For this review, take the finished solid that the model builds, in its own axes (mm). A direction names the side the tool comes from. Round coordinates to 2 decimals unless told otherwise and drop trailing zeros. Loops run counter-clockwise (first coordinate to the right, second up) from the corner with the lowest first, then second, coordinate; pieces in that order, holes last.
```python
from build123d import *

# Parameters (mm, degrees)
ESQUISSE1_R             = 20
BOSS_EXTRU_1_DEPTH      = 85
ESQUISSE6_R             = 8
ENL_V_MAT_EXTRU_1_DEPTH = 85
ESQUISSE7_R             = 11
ENL_V_MAT_EXTRU_2_DEPTH = 7
ESQUISSE11_W            = 3
ESQUISSE11_H            = 2


with BuildPart() as part:
    # Esquisse1 → Boss.-Extru.1 (new body)
    with BuildSketch(Plane(origin=(0, 0, 0), x_dir=(1, 0, 0), z_dir=(0, 1, 0))):
        with Locations(Location((0, 0, 0), (0, 0, 270))):
            Circle(ESQUISSE1_R)
    extrude(amount=BOSS_EXTRU_1_DEPTH)

    # Esquisse6 → Enlèv. mat.-Extru.1 (cut)
    with BuildSketch(Plane.XZ):
        with Locations(Location((0, 0, 0), (0, 0, 270))):
            Circle(ESQUISSE6_R)
    extrude(amount=-ENL_V_MAT_EXTRU_1_DEPTH, mode=Mode.SUBTRACT)

    # Esquisse7 → Enlèv. mat.-Extru.2 (cut)
    with BuildSketch(Plane.XZ):
        with Locations(Location((0, 0, 0), (0, 0, 270))):
            Circle(ESQUISSE7_R)
    enl_v_mat_extru_2 = extrude(amount=-ENL_V_MAT_EXTRU_2_DEPTH, mode=Mode.SUBTRACT)

    # Symétrie1: Enlèv. mat.-Extru.2 across plane
    add(enl_v_mat_extru_2.mirror(Plane.ZX.offset(42.5)), mode=Mode.SUBTRACT)

    # Esquisse11 → Révolution1 (revolve)
    with BuildSketch(Plane(origin=(0, 0, 0), x_dir=(0, 0, -1), z_dir=(1, 0, 0))):
        with Locations((21.485433731, 1)):
            Rectangle(ESQUISSE11_W, ESQUISSE11_H)
    r_volution1 = revolve(axis=Axis((0, 85, 0), (0, -1, 0)))

    # Symétrie2: Révolution1 across plane
    add(r_volution1.mirror(Plane.ZX.offset(42.5)))


solid = part.part
```
(1) For faces 1 (the cylindrical face through (15.535, 83.986, 16.941)), 2 (the flat face through (-20.3, 83, -1.8)), 3 (the cylindrical face through (-10.74, 3.45, 2.38)), 4 (the cylindrical face through (-10.74, 81.55, 2.38)), list the 3-axis set-ups (+Z, -Z, +X, -X, +Y, -Y) from which the entire face can be reached by the end or side of a thin tool; tool diameter is ignored.
(2) Add section C-C (y = 6). Give the boundary of the cut face in (x, z), plus the area to 3 significant figures.
(3) Add section D-D (z = -9.5). Give the boundary of the cut face in (x, y).
(4) Add section A-A (x = 0). Give the boundary of the cut face in (y, z).
(5) The part is to be moulded in two halves that separate along Z. For faces 5 (the flat face through (-8, 78, 2)), 6 (the flat face through (-10, 85, -5)), 7 (the cylindrical face through (-19.524, 41.933, -4.336)), say which applies: pulls with the +Z half, pulls with the -Z half, needs draft (parallel to the pull), parting line crosses it, or undercut.
(6) For L1, parallel to X at y = 5.25, z = 0; L2, parallel to X at y = 26, z = 0; L3, parallel to Y at x = -9, z = 4.5, list the stretches that pass through material, from the lowest coordinate up.
(7) Insertion check: pin 1 Ø2 at (x, z) = (-2, -12) entering from -Y; pin 2 Ø6 at (x, y) = (0, 41) entering from +Z; pin 3 Ø4 at (y, z) = (39, -14) entering from +X; pin 4 Ø6 at (x, y) = (-4.5, 18) entering from -Z. Each pin has a flat end and moves straight along its axis. Give the tip position at first contact, or say it passes through.
(8) Add section B-B (z = 0). Give the boundary of the cut face in (x, y), plus the area to 3 significant figures.
Outcome:
1. face 1: +Y, -Y
1. face 2: none
1. face 3: -Y
1. face 4: +Y
2. outline: circle Ø40 at (0, 0); hole circle Ø22 at (0, 0)
2. area: 877 mm2
3. outline: (-20.93, 0) - (-5.55, 0) - (-5.55, 7) - (5.55, 7) - (5.55, 0) - (20.93, 0) - (20.93, 2) - (17.6, 2) - (17.6, 83) - (20.93, 83) - (20.93, 85) - (5.55, 85) - (5.55, 78) - (-5.55, 78) - (-5.55, 85) - (-20.93, 85) - (-20.93, 83) - (-17.6, 83) - (-17.6, 2) - (-20.93, 2) - close
4. outline: (0, -22.99) - (2, -22.99) - (2, -20) - (83, -20) - (83, -22.99) - (85, -22.99) - (85, -11) - (78, -11) - (78, -8) - (7, -8) - (7, -11) - (0, -11) - close; (0, 11) - (7, 11) - (7, 8) - (78, 8) - (78, 11) - (85, 11) - (85, 22.99) - (83, 22.99) - (83, 20) - (2, 20) - (2, 22.99) - (0, 22.99) - close
5. face 5: undercut
5. face 6: needs draft
5. face 7: parting line crosses it
6. L1: x = -20 to -11, 11 to 20
6. L2: x = -20 to -8, 8 to 20
6. L3: y = 7 to 78
7. pin 1: stops at y = 0
7. pin 2: stops at z = 20
7. pin 3: stops at x = 16
7. pin 4: stops at z = -19.94
8. outline: (-22.99, 0) - (-11, 0) - (-11, 7) - (-8, 7) - (-8, 78) - (-11, 78) - (-11, 85) - (-22.99, 85) - (-22.99, 83) - (-20, 83) - (-20, 2) - (-22.99, 2) - close; (8, 7) - (11, 7) - (11, 0) - (22.99, 0) - (22.99, 2) - (20, 2) - (20, 83) - (22.99, 83) - (22.99, 85) - (11, 85) - (11, 78) - (8, 78) - close
8. area: 1,980 mm2
